```python
from build123d import *

# Parameters (mm, degrees)
SKETCH1_W           = 175
SKETCH1_H           = 139.7
BOSS_EXTRUDE1_DEPTH = 3.18
SKETCH2_R           = 1.5
SKETCH2_W           = 3.18
SKETCH2_H           = 59.975
CUT_EXTRUDE1_DEPTH  = 4.18
SKETCH3_R           = 1.59
CUT_EXTRUDE2_DEPTH  = 4.18
SKETCH4_R           = 1.59
CUT_EXTRUDE3_DEPTH  = 4.18
SKETCH5_W           = 91.926224914
SKETCH5_H           = 123.656630911
BOSS_EXTRUDE2_DEPTH = 3.18
SKETCH6_W           = 3.18
SKETCH6_H           = 19.75
CUT_EXTRUDE4_DEPTH  = 4.18
SKETCH8_W           = 25.560381265
SKETCH8_H           = 19.67928192
BOSS_EXTRUDE3_DEPTH = 3.18
SKETCH10_W          = 20
SKETCH10_H          = 2.468001363
BOSS_EXTRUDE4_DEPTH = 3.18
CUT_EXTRUDE5_DEPTH  = 4.18
SKETCH12_W          = 36.012104279
SKETCH12_H          = 43.960205632
CUT_EXTRUDE6_DEPTH  = 4.18
SKETCH13_W          = 16.174082381
SKETCH13_H          = 26.705141904
CUT_EXTRUDE7_DEPTH  = 4.18
SKETCH16_W          = 18.884338216
SKETCH16_H          = 121.056150973
SKETCH16_W_2        = 10.857087527
SKETCH16_H_2        = 35.437593219
SKETCH16_W_3        = 28.428801023
SKETCH16_H_3        = 14.001351757
SKETCH16_W_4        = 22.576937907
SKETCH16_H_4        = 16.729537969
BOSS_EXTRUDE6_DEPTH = 3.18
BOSS_EXTRUDE7_DEPTH = 3.18


with BuildPart() as part:
    # Sketch1 → Boss-Extrude1 (new body)
    with BuildSketch(Plane.XY):
        Rectangle(SKETCH1_W, SKETCH1_H)
    extrude(amount=BOSS_EXTRUDE1_DEPTH)

    # Sketch2 → Cut-Extrude1 (cut, through all)
    with BuildSketch(Plane.XY.offset(3.18)):
        with Locations((-85.5, 0)):
            Circle(SKETCH2_R)
        with Locations((85.5, 0)):
            Circle(SKETCH2_R)
        Polygon((-10, 69.85), (10, 69.85), (10, 66.67), (1.5, 66.67), (1.5, 62.67), (3.5, 62.67), (3.5, 59.67), (1.5, 59.67), (1.5, 56.67), (-1.5, 56.67), (-1.5, 59.67), (-3.5, 59.67), (-3.5, 62.67), (-1.5, 62.67), (-1.5, 66.67), (-10, 66.67), align=None)
        Polygon((-10, -69.85), (-10, -66.67), (-1.5, -66.67), (-1.5, -62.67), (-3.5, -62.67), (-3.5, -59.67), (-1.5, -59.67), (-1.5, -56.67), (1.5, -56.67), (1.5, -59.67), (3.5, -59.67), (3.5, -62.67), (1.5, -62.67), (1.5, -66.67), (10, -66.67), (10, -69.85), align=None)
        with Locations((-85.91, 39.8625)):
            Rectangle(SKETCH2_W, SKETCH2_H)
        with Locations((-85.91, -39.8625)):
            Rectangle(SKETCH2_W, SKETCH2_H)
        with Locations((85.91, -39.8625)):
            Rectangle(SKETCH2_W, SKETCH2_H)
        with Locations((85.91, 39.8625)):
            Rectangle(SKETCH2_W, SKETCH2_H)
        Polygon((-28.854904074, -66.67), (-20.334061159, -66.67), (-20.334061159, -69.85), (-40.334061159, -69.85), (-40.334061159, -66.67), (-31.854904074, -66.67), (-31.854904074, -62.67), (-33.77295002, -62.67), (-33.77295002, -59.67), (-31.854904074, -59.67), (-31.854904074, -56.85), (-28.854904074, -56.85), (-28.854904074, -59.67), (-26.77295002, -59.67), (-26.77295002, -62.67), (-28.854904074, -62.67), align=None)
    extrude(amount=-CUT_EXTRUDE1_DEPTH, mode=Mode.SUBTRACT)

    # Sketch3 → Cut-Extrude2 (cut, through all)
    with BuildSketch(Plane(origin=(0, 0, 0), x_dir=(-1, 0, 0), z_dir=(0, 0, -1))):
        with Locations((-35.67127699, -47.963396943)):
            Circle(SKETCH3_R)
        with Locations((-35.67127699, -30.777287406)):
            Circle(SKETCH3_R)
    extrude(amount=-CUT_EXTRUDE2_DEPTH, mode=Mode.SUBTRACT)

    # Sketch4 → Cut-Extrude3 (cut, through all)
    with BuildSketch(Plane(origin=(0, 0, 0), x_dir=(-1, 0, 0), z_dir=(0, 0, -1))):
        with Locations((-34.750723073, 53.780323187)):
            Circle(SKETCH4_R)
        with Locations((-34.750723073, 36.59421365)):
            Circle(SKETCH4_R)
        with Locations((36.249784221, 53.780323187)):
            Circle(SKETCH4_R)
        with Locations((36.249784221, 36.59421365)):
            Circle(SKETCH4_R)
        with Locations((35.983928162, -30.777287406)):
            Circle(SKETCH4_R)
        with Locations((35.983928162, -47.963396943)):
            Circle(SKETCH4_R)
        with Locations((-35.67127699, -30.777287406)):
            Circle(SKETCH4_R)
        with Locations((-35.67127699, -47.963396943)):
            Circle(SKETCH4_R)
    extrude(amount=-CUT_EXTRUDE3_DEPTH, mode=Mode.SUBTRACT)

    # Sketch5 → Boss-Extrude2 (add)
    with BuildSketch(Plane.XY.offset(3.18)):
        with Locations((-0.563564665, 5.553683182)):
            Rectangle(SKETCH5_W, SKETCH5_H)
    extrude(amount=-BOSS_EXTRUDE2_DEPTH)

    # Sketch6 → Cut-Extrude4 (cut, through all)
    with BuildSketch(Plane(origin=(0, 0, 0), x_dir=(-1, 0, 0), z_dir=(0, 0, -1))):
        with Locations((-25.21, 0.03599429)):
            Rectangle(SKETCH6_W, SKETCH6_H)
        with Locations((13.073612417, 0)):
            Rectangle(SKETCH6_W, SKETCH6_H)
    extrude(amount=-CUT_EXTRUDE4_DEPTH, mode=Mode.SUBTRACT)

    # Sketch8 → Boss-Extrude3 (add)
    with BuildSketch(Plane(origin=(0, 0, 0), x_dir=(-1, 0, 0), z_dir=(0, 0, -1))):
        with Locations((-2.780190633, -60.01035904)):
            Rectangle(SKETCH8_W, SKETCH8_H)
    extrude(amount=-BOSS_EXTRUDE3_DEPTH)

    # Sketch10 → Boss-Extrude4 (add)
    with BuildSketch(Plane(origin=(0, 0, 0), x_dir=(-1, 0, 0), z_dir=(0, 0, -1))):
        with Locations((0, 68.615999319)):
            Rectangle(SKETCH10_W, SKETCH10_H)
    extrude(amount=-BOSS_EXTRUDE4_DEPTH)

    # Sketch11 → Cut-Extrude5 (cut, through all)
    with BuildSketch(Plane(origin=(0, 0, 0), x_dir=(-1, 0, 0), z_dir=(0, 0, -1))):
        Polygon((20.793148035, 66.67), (29.479057969, 66.67), (29.479057969, 62.67), (27.293148035, 62.67), (27.293148035, 59.67), (29.479057969, 59.67), (29.479057969, 56.85), (32.479057969, 56.85), (32.479057969, 59.67), (34.293148035, 59.67), (34.293148035, 62.67), (32.479057969, 62.67), (32.479057969, 66.67), (40.793148035, 66.67), (40.793148035, 69.85), (20.793148035, 69.85), align=None)
    extrude(amount=-CUT_EXTRUDE5_DEPTH, mode=Mode.SUBTRACT)

    # Sketch12 → Cut-Extrude6 (cut, through all)
    with BuildSketch(Plane(origin=(0, 0, 0), x_dir=(-1, 0, 0), z_dir=(0, 0, -1))):
        with Locations((58.477018613, 4.914539536)):
            Rectangle(SKETCH12_W, SKETCH12_H)
    extrude(amount=-CUT_EXTRUDE6_DEPTH, mode=Mode.SUBTRACT)

    # Sketch13 → Cut-Extrude7 (cut, through all)
    with BuildSketch(Plane(origin=(0, 0, 0), x_dir=(-1, 0, 0), z_dir=(0, 0, -1))):
        with Locations((-9.848843291, 0)):
            Rectangle(SKETCH13_W, SKETCH13_H)
    extrude(amount=-CUT_EXTRUDE7_DEPTH, mode=Mode.SUBTRACT)

    # Sketch16 → Boss-Extrude6 (add)
    with BuildSketch(Plane(origin=(0, 0, 0), x_dir=(-1, 0, 0), z_dir=(0, 0, -1))):
        with Locations((-31.859595144, -9.321924514)):
            Rectangle(SKETCH16_W, SKETCH16_H)
        with Locations((12.113243242, -1.915189585)):
            Rectangle(SKETCH16_W_2, SKETCH16_H_2)
        with Locations((31.756187516, -62.849324122)):
            Rectangle(SKETCH16_W_3, SKETCH16_H_3)
        with Locations((32.081616989, 61.485231016)):
            Rectangle(SKETCH16_W_4, SKETCH16_H_4)
    extrude(amount=-BOSS_EXTRUDE6_DEPTH)

    # Sketch17 → Boss-Extrude7 (add)
    with BuildSketch(Plane(origin=(0, 0, 0), x_dir=(-1, 0, 0), z_dir=(0, 0, -1))):
        Polygon((-87.5, -69.85), (84.32, -69.85), (84.32, 69.85), (-87.5, 69.85), (-87.5, 74.493800826), (84.32, 74.493800826), (87.808220565, 74.493800826), (87.808220565, -69.85), (87.808220565, -75.025003811), (84.32, -75.025003811), (-87.5, -75.025003811), align=None)
    extrude(amount=-BOSS_EXTRUDE7_DEPTH)


solid = part.part
```
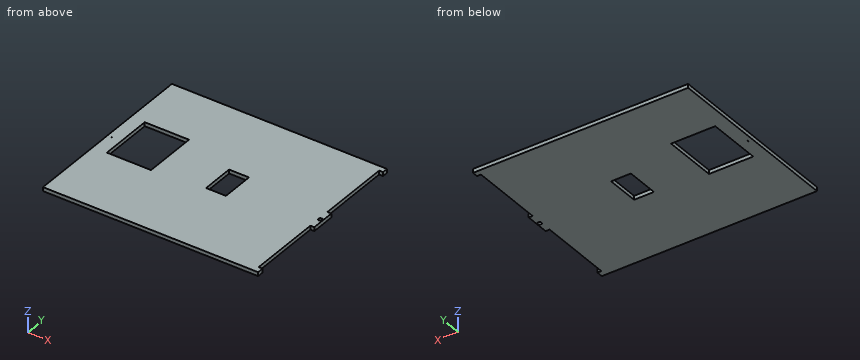
Geometry check sheet. Reference: the model listing, model coordinates, mm. Give positions to 0.01 mm unless a question says otherwise; leave off trailing zeros. Write each loop counter-clockwise with the first axis right and the second up, starting at its lowest first coordinate (ties: lowest second). Pieces come first, ordered by that corner, then holes.
1) Section check A-A, the plane x = -46. Record the boundary of the cut face in (y, z) (3 decimals).
2) Section check C-C, the plane y = 38. Record the boundary of the cut face in (x, z), and give its area (3 significant figures).
3) Section check B-B, the plane z = 2.55. Record the boundary of the cut face in (x, y) (3 decimals), and give its area (3 significant figures).
4) Material ranges on L1, parallel to Y at x = 85.5, z = 1.9 (3 decimals); L2, parallel to X at y = -12.5, z = 2.65; L3, parallel to X at y = 25, z = 0.7, recorded low to high.
Computed:
1. outline: (-75.025, 0) - (-17.066, 0) - (-17.066, 3.18) - (-75.025, 3.18) - close; (26.895, 0) - (74.494, 0) - (74.494, 3.18) - (26.895, 3.18) - close
2. outline: (-87.81, 0) - (84.32, 0) - (84.32, 3.18) - (-87.81, 3.18) - close
2. area: 547 mm2
3. outline: (-87.808, -75.025) - (87.5, -75.025) - (87.5, -69.85) - (84.32, -69.85) - (84.32, -9.875) - (87.5, -9.875) - (87.5, 9.875) - (84.32, 9.875) - (84.32, 69.85) - (87.5, 69.85) - (87.5, 74.494) - (-87.808, 74.494) - close; hole (-84.32, -0.926) arc R1.5 ccw to (-84.32, 0.926) - close; hole (-76.483, -17.066) - (-40.471, -17.066) - (-40.471, 26.895) - (-76.483, 26.895) - close; hole (1.762, -13.353) - (17.936, -13.353) - (17.936, 13.353) - (1.762, 13.353) - close; hole circle Ø3 at (85.5, 0)
3. area: 23,800 mm2
4. L1: y = -75.025 to -69.85, -9.875 to -1.5, 1.5 to 9.875, 69.85 to 74.494
4. L2: x = -87.81 to -76.48, -40.47 to 1.76, 17.94 to 84.32
4. L3: x = -87.81 to -76.48, -40.47 to 84.32
